Geometry: final body of the model. Coordinates: model frame, mm. Coordinates: 2 decimals unless noted, no trailing zeros. Order: outer loops, then holes, each group sorted by start corner. A loop starts at its lowest first (then second) coordinate and runs counter-clockwise, first axis right, second up. Notation, with made-up numbers: (-2, -39) - (6, -39) arc R24 ccw to (6, -24) - close; hole circle Ø11 at (76, -26.75). An arc over 180 degrees is marked (long way). Use a Markdown table: item, result. Add a question column.
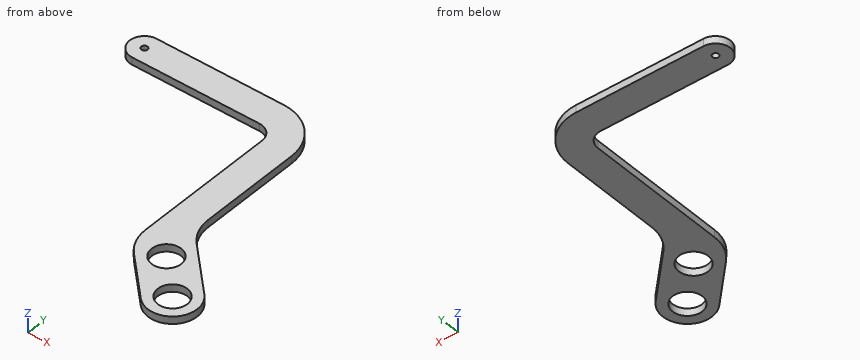
Autodesk Inventor part; units mm, degrees
ref_plane "YZ Plane" through (0, 0, 0) normal (1, 0, 0) x (0, 1, 0)
ref_plane "XZ Plane" through (0, 0, 0) normal (0, 1, 0) x (-1, 0, 0)
ref_plane "XY Plane" through (0, 0, 0) normal (0, 0, 1) x (1, 0, 0)
sketch "Sketch1" plane through (0, 0, 0) normal (0, 0, 1) x (1, 0, 0)
  circle A0 centre (0, 0) radius 9.525
  line L0 (0, 9.525) -> (81.915, 9.525)
  arc A1 (110.49, -19.05) -> (81.915, 9.525) centre (81.915, -19.05) ccw
  line L1 (110.49, -19.05) -> (110.49, -94.7987)
  line L2 (110.49, -94.7987) -> (146.411, -130.7197)
  arc A2 (123.9604, -153.1704) -> (146.411, -130.7197) centre (135.1857, -141.9451) ccw
  line L3 (123.9604, -153.1704) -> (91.44, -120.65)
  line L4 (91.44, -120.65) -> (91.44, -19.05)
  arc A3 (91.44, -19.05) -> (81.915, -9.525) centre (81.915, -19.05) ccw
  line L5 (81.915, -9.525) -> (0, -9.525)
  circle A4 centre (135.1857, -141.9451) radius 9.525
  circle A5 centre (112.7351, -119.4944) radius 9.525
  line L6 (135.1857, -141.9451) -> (112.7351, -119.4944) construction
  dimension "d0" = 19.05
  dimension "d1" = 9.525
  dimension "d4" = 91.44
  dimension "d5" = 101.6
  dimension "d6" = 31.75
  dimension "d7" = 50.8
  dimension "d8" = 19.05
  dimension "d9" = 19.05
  dimension "d10" = 31.75
  dimension "d11" = 135
extrude "Extrusion1" add sketch "Sketch1" along normal blind 4.7625
sketch "Sketch2" plane through (0, 0, 4.7625) normal (0, 0, 1) x (1, 0, 0)
  arc A0 (0, 9.525) -> (0, -9.525) centre (0, 0) ccw construction
hole "Hole1" at (0, 0, 4.7625) direction (0, 0, -1) diameter 3.9624 end through all
fillet "Fillet1" radius 25.4 2 edges at (110.49, -94.7987, 2.3813) (91.44, -120.65, 2.3813)
equation "\"BendRadius\" = Thickness"
equation "\"BendReliefWidth\" = Thickness"
equation "\"BendReliefDepth\" = 0.5 * Thickness"
equation "\"CornerReliefSize\" = 4 * Thickness"
equation "\"MinimumRemnant\" = 2 * Thickness"
equation "\"TransitionRadius\" = BendRadius"
equation "\"JacobiRadiusSize\" = BendRadius"
equation "\"GapSize\" = Thickness"
properties part number "ARM,KICKER"
1) Section query A-A (z = 2.05). Return the cut outline in (x, y) (3 decimals).
2) Line query: line 1 (X direction, y = 0, z = 3) (3 decimals); line 2 (Y direction, x = 7.5, z = 1.4) (3 decimals); line 3 (Y direction, x = 0, z = 2.1) (3 decimals). Output: solid intervals per line, ascending. Write a range as from..to.
3) Section query D-D (y = -65.5). Return the cut outline in (x, z), and give its area (3 significant figures).
4) Section query B-B (x = 141.5). Return the cut outline in (y, z), and give its area (3 significant figures).
5) First-contact query: pin 1 (22 mm diameter, centred on x = 135.19, y = -141.95, fed in from +Z); pin 2 (1 mm diameter, centred on x = 86, z = 2.5, fed in from -Y); pin 3 (2 mm diameter, centred on y = -102, z = 1.5, fed in from +X); pin 4 (1.4 mm diameter, centred on y = -50, z = 2, fed in from +X). Flat tips, straight axial feed; report the tip coordinate or a pass-through.
6) Section query C-C (y = 0). Return the cut outline in (x, z) (1 decimal), and give its area (3 significant figures).
From the geometry:
| question | item | result |
|---|---|---|
| 1 | outline | (0, -9.525) - (81.915, -9.525) arc R9.525 cw to (91.44, -19.05) - (91.44, -110.129) arc R25.4 ccw to (98.879, -128.089) - (123.96, -153.17) arc R15.875 ccw to (146.411, -130.72) - (117.929, -102.238) arc R25.4 cw to (110.49, -84.278) - (110.49, -19.05) arc R28.575 ccw to (81.915, 9.525) - (0, 9.525) arc R9.525 ccw to start; hole circle Ø3.962 at (0, 0); hole circle Ø19.05 at (112.735, -119.494); hole circle Ø19.05 at (135.186, -141.945) |
| 2 | line 1 | x = -9.525..-1.981, 1.981..103.214 |
| 2 | line 2 | y = -9.525..9.525 |
| 2 | line 3 | y = -9.525..-1.981, 1.981..9.525 |
| 3 | outline | (91.44, 0) - (110.49, 0) - (110.49, 4.76) - (91.44, 4.76) - close |
| 3 | area | 90.7 mm^2 |
| 4 | outline | (-156.51, 0) - (-149.08, 0) - (-149.08, 4.76) - (-156.51, 4.76) - close; (-134.81, 0) - (-125.81, 0) - (-125.81, 4.76) - (-134.81, 4.76) - close |
| 4 | area | 78.3 mm^2 |
| 5 | pin 1 | stops at z = 4.76 |
| 5 | pin 2 | stops at y = -10.7 |
| 5 | pin 3 | stops at x = 118.69 |
| 5 | pin 4 | stops at x = 110.49 |
| 6 | outline | (-9.5, 0) - (-2, 0) - (-2, 4.8) - (-9.5, 4.8) - close; (2, 0) - (103.2, 0) - (103.2, 4.8) - (2, 4.8) - close |
| 6 | area | 518 mm^2 |
